Could you check a few things on this model? Use its own coordinates, in mm. Face numbers are marked on the shaded views. Round coordinates to 2 decimals unless told otherwise and drop trailing zeros. Loops run counter-clockwise (first coordinate to the right, second up) from the corner with the lowest first, then second, coordinate; pieces in that order, holes last. Notation, with made-up numbers: M 44.25,-1 L 68.25,-1 A12 cw 68.25,5 Z; hole C 20,-11 d1. An arc over 180 degrees is marked long. Answer in a Markdown table with one row per item.
```python
from build123d import *

# Parameters (mm, degrees)
SKETCH_R      = 38
PAD_DEPTH     = 2
SKETCH001_R   = 36.75
SKETCH001_R_2 = 35
PAD001_DEPTH  = 22.6
SKETCH002_R   = 5.191137
SKETCH002_R_2 = 2.55
PAD002_DEPTH  = 10
FILLET_R      = 1
FILLET001_R   = 0.5


with BuildPart() as part:
    # Sketch → Pad (new body)
    with BuildSketch(Plane.XY):
        Circle(SKETCH_R)
    extrude(amount=PAD_DEPTH)

    # Sketch001 → Pad001 (new body)
    with BuildSketch(Plane.XY.offset(2)):
        Circle(SKETCH001_R)
        Circle(SKETCH001_R_2, mode=Mode.SUBTRACT)
    extrude(amount=PAD001_DEPTH)

    # Sketch002 → Pad002 (new body)
    with BuildSketch(Plane.XY.offset(2)):
        Circle(SKETCH002_R)
        Circle(SKETCH002_R_2, mode=Mode.SUBTRACT)
    extrude(amount=PAD002_DEPTH)

    # Fillet
    fillet_edges = [part.edges().sort_by_distance(p)[0] for p in [
        (5.191137, 0, 7),
        (-5.191137, 0, 12),
    ]]
    fillet(fillet_edges, radius=FILLET_R)

    # Fillet001
    fillet001_edges = [part.edges().sort_by_distance(p)[0] for p in [
        (-36.75, 0, 24.6),
        (-35, 0, 24.6),
    ]]
    fillet(fillet001_edges, radius=FILLET001_R)


solid = part.part
```
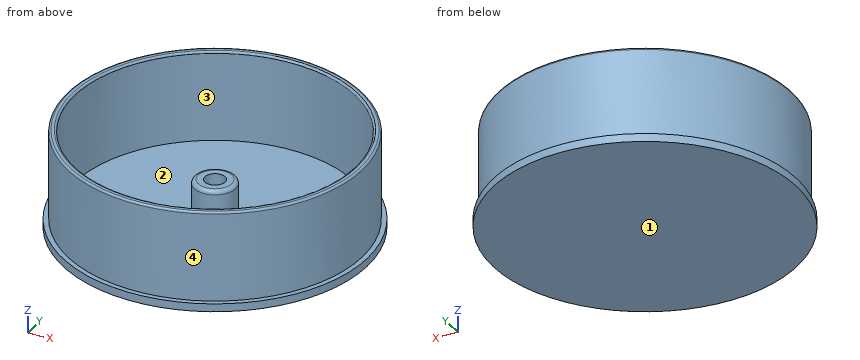
1) I want a section at A-A, the plane z = 8.5. Please give me the cut outline in (x, y).
Computed:
| item | result |
|---|---|
| outline | C 0,0 d73.5; C 0,0 d10.38; hole C 0,0 d70; hole C 0,0 d5.1 |
2) Will these pins go through, and if not, where does the flat tip stop? P1, Ø2.5, axis at x = 1, y = 0, coming from the +Z side; P2, Ø5, axis at y = 14, z = 11, coming from the -X side; P3, Ø4, axis at x = 15, z = 6, coming from the +Y side.
Computed:
| item | result |
|---|---|
| P1 | stops at z = 2 |
| P2 | stops at x = -34.9 |
| P3 | stops at y = 34.37 |
3) I want a section at B-B, the plane x = 0. Please give me the cut outline in (y, z), plus the area to 3 significant figures.
Computed:
| item | result |
|---|---|
| outline | M -38,0 L 38,0 L 38,2 L 36.75,2 L 36.75,24.1 A0.5 ccw 36.25,24.6 L 35.5,24.6 A0.5 ccw 35,24.1 L 35,2 L 5.19,2 L 5.19,11 A1 ccw 4.19,12 L 2.55,12 L 2.55,2 L -2.55,2 L -2.55,12 L -4.19,12 A1 ccw -5.19,11 L -5.19,2 L -35,2 L -35,24.1 A0.5 ccw -35.5,24.6 L -36.25,24.6 A0.5 ccw -36.75,24.1 L -36.75,2 L -38,2 Z |
| area | 283 mm² |
4) I need wall thicknesses on line 1 (Y direction, x = 0, z = 15.75); line 2 (Y direction, x = 0, z = 7.25); line 3 (Z direction, x = -0.5, y = -10). Which ranges of each line are inside material? Lowest first, please.
Computed:
| item | result |
|---|---|
| line 1 | y = -36.75 to -35, 35 to 36.75 |
| line 2 | y = -36.75 to -35, -5.19 to -2.55, 2.55 to 5.19, 35 to 36.75 |
| line 3 | z = 0 to 2 |
5) If we mould it in two halves opening along X, with no side actions, what happens to the marked faces 1, 2, 3 and 4? For each: released by +X, released by -X, zero draft, split by the parting line, or undercut.
Computed:
| item | result |
|---|---|
| face 1 | zero draft |
| face 2 | undercut |
| face 3 | undercut |
| face 4 | split by the parting line |
6) I want a section at D-D, the plane z = 20.5. Please give me the cut outline in (x, y), plus the area to 3 significant figures.
Computed:
| item | result |
|---|---|
| outline | C 0,0 d73.5; hole C 0,0 d70 |
| area | 394 mm² |
